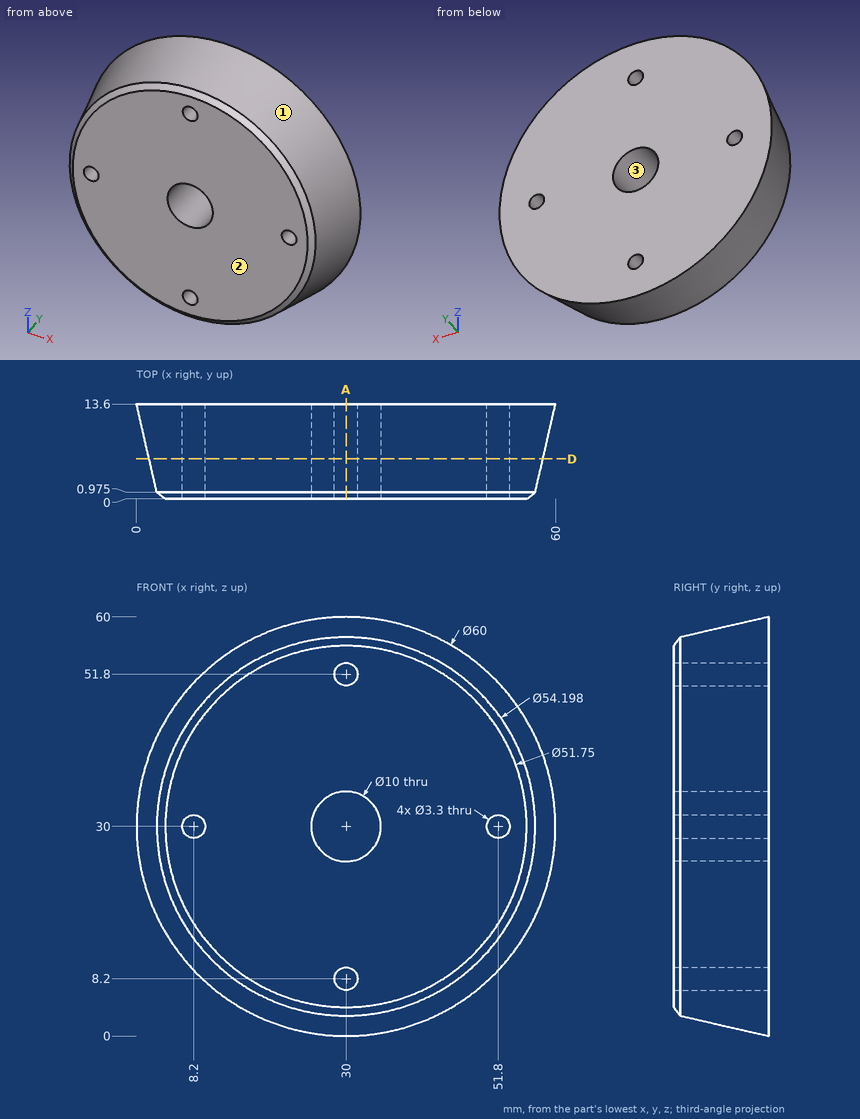
Design review of the part shown in the three views and the two pictorial views. Dimensions are in mm from the part's minimum x, y and z. Round coordinates to 2 decimals unless told otherwise and drop trailing zeros. Loops run counter-clockwise (first coordinate to the right, second up) from the corner with the lowest first, then second, coordinate; pieces in that order, holes last. Notation, with made-up numbers: (32.25, 24) - (91.25, 24) arc R12 cw to (91.25, 46) - close; hole circle Ø7 at (77.5, 31.25). An arc over 180 degrees is marked (long way). Write each question's results on one line, items separated by ' | '. Start each with the question number.
Q1. Take a section at D-D on y = 5.75. Give the boundary of the cut face in (x, z), plus the area to 4 significant figures.
Q2. Take a section at A-A on x = 30. Give the number of separate pieces and of enclosed holes in the cut face, plus the area to 3 significant figures.
Q3. Wall thickness on line 1 along Z through (x, y) = (30, 4.75); line 2 along Z through (x, y) = (30, 3.5); line 3 along X through (y, z) = (10, 7) (1 decimal): over which ranges is each line inside the solid? List them lowest first. Write a range as [from, to].
Q4. Draft analysis for pull direction X (two halves, no side actions). For the marked faces 1, 2 and 3, state which applies: pulls with the +X half, pulls with the -X half, needs draft (parallel to the pull), parting line crosses it, or undercut.
Q5. Insertion check: P1, Ø3, axis at y = 1.5, z = 50, coming from the -X side (1 decimal); P2, Ø3, axis at y = 9.5, z = 20.5, coming from the +X side; P3, Ø1.5, axis at x = 54, y = 6.5, coming from the -Z side (1 decimal). Each pin has a flat end and moves straight along its axis. Give the tip position at first contact, or say it passes through.
Data:
1) outline: circle Ø56.39 at (30, 30); hole circle Ø3.3 at (8.2, 30); hole circle Ø10 at (30, 30); hole circle Ø3.3 at (30, 8.2); hole circle Ø3.3 at (30, 51.8); hole circle Ø3.3 at (51.8, 30) | area: 2,385 mm²
2) separate pieces: 4 | enclosed holes: 0 | area: 547 mm²
3) line 1: z = [2.03, 6.55], [9.85, 25], [35, 50.15], [53.45, 57.97] | line 2: z = [2.32, 6.55], [9.85, 25], [35, 50.15], [53.45, 57.68] | line 3: x = [12.1, 28.9], [31.1, 47.9]
4) face 1: parting line crosses it | face 2: needs draft | face 3: undercut
5) P1: stops at x = 10 | P2: stops at x = 58.06 | P3: stops at z = 13.7
